Could you check a few things on this drawing? It's one solid part, dimensions in mm from its lowest x, y, z. Give positions to 0.01 mm unless a question says otherwise; leave off trailing zeros. Loops run counter-clockwise (first coordinate to the right, second up) from the corner with the lowest first, then second, coordinate; pieces in that order, holes last. Notation, with made-up numbers: (-19.5, 5) - (21.5, 5) arc R13 ccw to (21.5, 26) - close; hole circle Ø10 at (59.5, -38). An arc over 180 degrees is marked (long way). Return JSON: item names as keys, results as strings. Group by question number.
(1) If we section it at D-D (x = 31): Please give me the cut outline in (y, z) (1 decimal), then the cut area to 3 significant figures.
(2) If we section it at B-B (z = 0.6): Please give me the cut outline in (x, y) (1 decimal).
(3) If we section it at A-A (y = 8.5): Please give me the cut outline in (x, z) (1 decimal).
(4) If we section it at C-C (y = 16.5): Please give me the cut outline in (x, z) (1 decimal).
(5) I need wall thicknesses on probe 1 along X at (y, z) = (15.25, 1.15); probe 2 along X at (y, z) = (15.5, 0.5) (1 decimal); probe 3 along Y at (x, z) = (10.5, 1.9). Which ranges of each line are inside material? Lowest first, please. Write a range as [from, to].
(6) For P1, Ø1, axis at y = 15, z = 1.5, coming from the +X side; P2, Ø1, axis at y = 16.5, z = 1, coming from the -X side; P3, Ø2.5, axis at x = 39.11, y = 11.25, coming from the -Z side; P4, Ø0.6, axis at x = 11.5, z = 1, coming from the +Y side, each with a flat end and sliding along its axis, tell me the tip position at first contact or that it passes through.
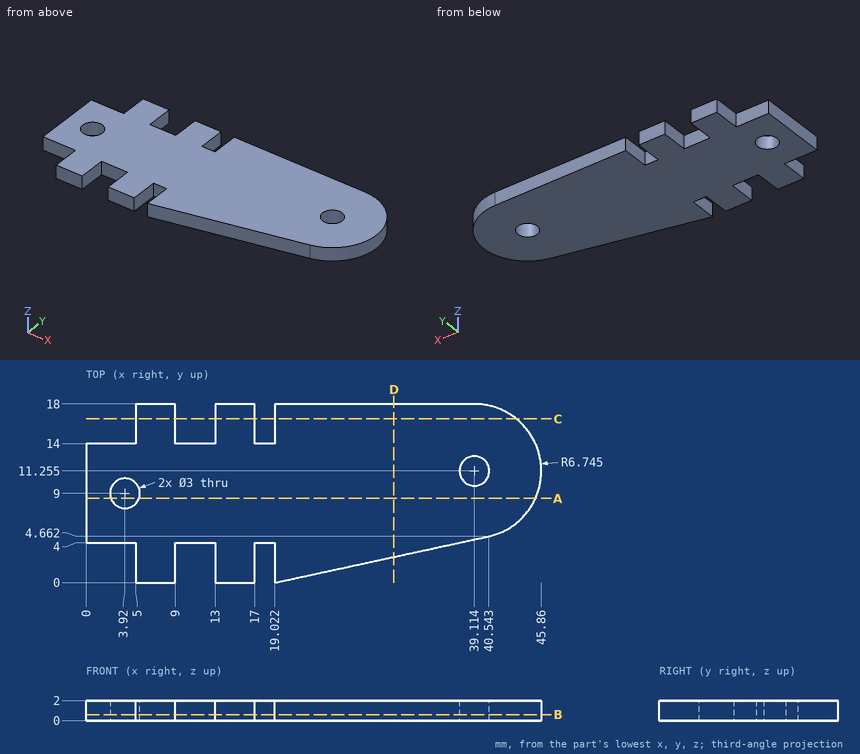
Values:
{
 "1": {"outline": "(2.6, 0) - (18, 0) - (18, 2) - (2.6, 2) - close", "area": "30.8 mm2"},
 "2": {"outline": "(0, 4) - (5, 4) - (5, 0) - (9, 0) - (9, 4) - (13, 4) - (13, 0) - (17, 0) - (17, 4) - (19, 4) - (19, 0) - (40.5, 4.7) arc R6.7 ccw to (39.1, 18) - (19, 18) - (19, 14) - (17, 14) - (17, 18) - (13, 18) - (13, 14) - (9, 14) - (9, 18) - (5, 18) - (5, 14) - (0, 14) - close; hole circle Ø3 at (3.9, 9); hole circle Ø3 at (39.1, 11.3)"},
 "3": {"outline": "(0, 0) - (2.5, 0) - (2.5, 2) - (0, 2) - close; (5.3, 0) - (45.3, 0) - (45.3, 2) - (5.3, 2) - close"},
 "4": {"outline": "(5, 0) - (9, 0) - (9, 2) - (5, 2) - close; (13, 0) - (17, 0) - (17, 2) - (13, 2) - close; (19, 0) - (43.4, 0) - (43.4, 2) - (19, 2) - close"},
 "5": {"probe 1": "[5, 9], [13, 17], [19.02, 44.55]", "probe 2": "[5, 9], [13, 17], [19, 44.4]", "probe 3": "[4, 14]"},
 "6": {"P1": "x = 45.03", "P2": "x = 5", "P3": "through", "P4": "y = 14"}
}
